```python
from build123d import *

# Parameters (mm, degrees)
BOSS_EXTRU_1_DEPTH      = 30
ESQUISSE2_R             = 2.5
ESQUISSE2_R_2           = 1
ENL_V_MAT_EXTRU_1_DEPTH = 73.427135799
ESQUISSE3_R             = 7
ENL_V_MAT_EXTRU_2_DEPTH = 2
ESQUISSE4_R             = 1
ENL_V_MAT_EXTRU_3_DEPTH = 71.503120498
CONG_2_R                = 1


with BuildPart() as part:
    # Esquisse1 → Boss.-Extru.1 (new body)
    with BuildSketch(Plane(origin=(0, 0, 0), x_dir=(0, 0, -1), z_dir=(1, 0, 0))):
        Polygon((0, 0), (0, 30), (5, 30), (5, 5), (58.7, 5), (58.7, 0), align=None)
    extrude(amount=BOSS_EXTRU_1_DEPTH)

    # Esquisse2 → Enl_v. mat.-Extru.1 (cut, through all)
    with BuildSketch(Plane.XY):
        with BuildLine():
            Line((30, 30), (15, 30))
            ThreePointArc((15, 30), (21.259063707, 28.04566866), (25.294075712, 22.877113002))
            Line((25.294075712, 22.877113002), (30, 5))
            Line((30, 5), (30, 30))
        make_face()
        with BuildLine():
            Line((0, 30), (0, 5))
            Line((0, 5), (4.705924288, 22.877113002))
            ThreePointArc((4.705924288, 22.877113002), (8.740936293, 28.04566866), (15, 30))
            Line((15, 30), (0, 30))
        make_face()
        with Locations((15, 19)):
            Circle(ESQUISSE2_R)
        with Locations((24, 19)):
            Circle(ESQUISSE2_R_2)
        with Locations((15, 10)):
            Circle(ESQUISSE2_R_2)
        with Locations((6, 19)):
            Circle(ESQUISSE2_R_2)
        with Locations((15, 28)):
            Circle(ESQUISSE2_R_2)
    extrude(amount=-ENL_V_MAT_EXTRU_1_DEPTH, mode=Mode.SUBTRACT)

    # Esquisse3 → Enl_v. mat.-Extru.2 (cut)
    with BuildSketch(Plane(origin=(0, 0, -5), x_dir=(-1, 0, 0), z_dir=(0, 0, -1))):
        with Locations(Location((-15, 19, 0), (0, 0, 90))):
            Circle(ESQUISSE3_R)
    extrude(amount=-ENL_V_MAT_EXTRU_2_DEPTH, mode=Mode.SUBTRACT)

    # Esquisse4 → Enl_v. mat.-Extru.3 (cut, through all)
    with BuildSketch(Plane(origin=(0, 5, 0), x_dir=(1, 0, 0), z_dir=(0, 1, 0))):
        with Locations(Location((3, 10.37, 0), (0, 0, 270))):
            Circle(ESQUISSE4_R)
        with Locations(Location((27, 10.37, 0), (0, 0, 90))):
            Circle(ESQUISSE4_R)
        with Locations(Location((27, 53.33, 0), (0, 0, 270))):
            Circle(ESQUISSE4_R)
        with Locations(Location((3, 53.33, 0), (0, 0, 90))):
            Circle(ESQUISSE4_R)
        with Locations(Location((3, 31.85, 0), (0, 0, 270))):
            Circle(ESQUISSE4_R)
        with Locations(Location((27, 31.85, 0), (0, 0, 90))):
            Circle(ESQUISSE4_R)
    extrude(amount=-ENL_V_MAT_EXTRU_3_DEPTH, mode=Mode.SUBTRACT)

    # Cong_2
    cong_2_edges = [part.edges().sort_by_distance(p)[0] for p in [
        (15, 5, -5),
    ]]
    fillet(cong_2_edges, radius=CONG_2_R)


solid = part.part
```
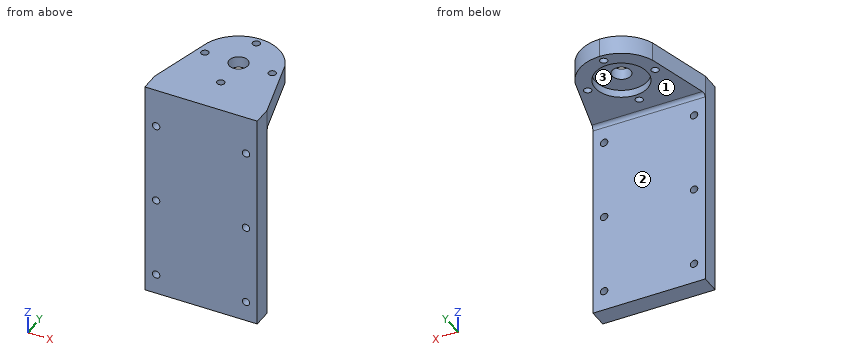
CAD build for the part. Positions are in the model's coordinates, mm. Face numbers are marked on the shaded views. Round coordinates to 2 decimals unless told otherwise and drop trailing zeros. Write each loop counter-clockwise with the first axis right and the second up, starting at its lowest first coordinate (ties: lowest second). Pieces come first, ordered by that corner, then holes. Notation, with made-up numbers: (34, 59.25) -> (61, 59.25) arc R24 ccw to (61, 92.25) -> close; hole circle Ø2 at (-23.5, -11). An arc over 180 degrees is marked (long way). Answer in a Markdown table with one row per item. Add a question column.
Item 1: Saw through at D-D, the plane z = -38. Write the cut outline in (x, y), then the cut area to 3 significant figures.
Item 2: Drill centre lines: line 1 (X direction, y = 1.3, z = -53.33); line 2 (Z direction, x = 26, y = 11.5); line 3 (Y direction, x = 25.5, z = -15). Where is each one in solid material? Low to high. Write a range as from..to.
Item 3: Saw through at B-B, the plane y = 10. Write the cut outline in (x, z), then the cut area to 3 significant figures.
Item 4: Drop flat-ended pins along their axis: pin 1 Ø12 at (y, z) = (15, -29.5) entering from +X; pin 2 Ø2.5 at (x, y) = (15, 28) entering from -Z; pin 3 Ø12 at (x, z) = (23, -35.5) entering from +Y. Give the stop position or say it passes through.
Item 5: Mould opens along Y. For the marked faces 1, 2 and 3 say: pulls with the +Y half, pulls with the -Y half, needs draft (parallel to the pull), parting line crosses it, or undercut.
Item 6: Saw through at C-C, the plane x = 27. Write the cut outline in (y, z), then the cut area to 3 significant figures.
Item 7: Saw through at A-A, the plane z = -10.37. Write the cut outline in (x, y).
Findings below:
| question | item | result |
|---|---|---|
| 1 | outline | (0, 0) -> (30, 0) -> (30, 5) -> (0, 5) -> close |
| 1 | area | 150 mm^2 |
| 2 | line 1 | x = 0..2, 4..26, 28..30 |
| 2 | line 2 | z = -5..0 |
| 2 | line 3 | y = 0..5 |
| 3 | outline | (1.32, -5) -> (14, -5) -> (14, 0) -> (1.32, 0) -> close; (16, -5) -> (28.68, -5) -> (28.68, 0) -> (16, 0) -> close |
| 3 | area | 127 mm^2 |
| 4 | pin 1 | passes through |
| 4 | pin 2 | stops at z = -5 |
| 4 | pin 3 | stops at y = 5 |
| 5 | face 1 | needs draft |
| 5 | face 2 | pulls with the +Y half |
| 5 | face 3 | undercut |
| 6 | outline | (0, -58.7) -> (5, -58.7) -> (5, -54.33) -> (0, -54.33) -> close; (0, -52.33) -> (5, -52.33) -> (5, -32.85) -> (0, -32.85) -> close; (0, -30.85) -> (5, -30.85) -> (5, -11.37) -> (0, -11.37) -> close; (0, -9.37) -> (5, -9.37) -> (5, -6) arc R1 cw to (6, -5) -> (16.4, -5) -> (16.4, 0) -> (0, 0) -> close |
| 6 | area | 321 mm^2 |
| 7 | outline | (0, 0) -> (2, 0) -> (2, 5) -> (0, 5) -> close; (4, 0) -> (26, 0) -> (26, 5) -> (4, 5) -> close; (28, 0) -> (30, 0) -> (30, 5) -> (28, 5) -> close |
